from build123d import *

# Parameters (mm, degrees)
F0_W    = 7
F0_H    = 11
F0_W_2  = 5
F0_H_2  = 15
F0_W_3  = 20
F0_H_3  = 7
F2_SIZE = 1.99999


# Not quite as in the source:
# - a fillet or chamfer is up to 0.001 mm smaller than in the source, because OpenCascade refuses the exact size


with BuildPart() as f1:
    # F0 (on Front) → F1 (revolve)
    with BuildSketch(Plane.XZ):
        Polygon((33, 0), (0, 0), (0, -13), (33, -13), (33, -11), align=None)
        with Locations((36.5, -5.5)):
            Rectangle(F0_W, F0_H)
        Polygon((49, 0), (40, 0), (40, -11), (40, -17), (49, -17), (49, -15), align=None)
        with Locations((51.5, -7.5)):
            Rectangle(F0_W_2, F0_H_2)
        Polygon((63, 0), (54, 0), (54, -15), (54, -17), (63, -17), (63, -9), align=None)
        Polygon((95, 0), (63, 0), (63, -9), (95, -9), (95, -7), align=None)
        with Locations((105, -3.5)):
            Rectangle(F0_W_3, F0_H_3)
    revolve(axis=Axis((51.5, 0, 0), (1, 0, 0)))

    # F2 (size 2 in the source; OpenCascade refuses exactly that, so slightly less here)
    f2_edges = [f1.edges().sort_by_distance(p)[0] for p in [
        (0, 0, 13),
        (33, 0, 13),
        (16.5, 0, -13),
        (40, 0, 17),
        (49, 0, 17),
        (54, 0, 17),
        (63, 0, 17),
        (95, 0, 9),
        (115, 0, 7),
    ]]
    chamfer(f2_edges, length=F2_SIZE)


solid = f1.part
Could you check a few things on this model? Use its own coordinates, in mm. A direction names the side the tool comes from. Give positions to 0.01 mm unless a question says otherwise; leave off trailing zeros. Order: outer loops, then holes, each group sorted by start corner. A loop starts at its lowest first (then second) coordinate and runs counter-clockwise, first axis right, second up. Notation, with made-up numbers: (26, 48.25) - (73, 48.25) arc R19 cw to (73, 79.25) - close; hole circle Ø5 at (6.25, 40.5). An arc over 180 degrees is marked (long way). One line per item, written item: value. Start each with the question number.
1. Imagine slicing it at A-A on x = 104. List the corners of the cut face in (y, z) for me.
2. Imagine slicing it at B-B on x = 18. List the corners of the cut face in (y, z) for me, plus the area to 3 significant figures.
3. If I drill on probe 1 along X at (y, z) = (-7, 14.5); probe 2 along X at (y, z) = (9, 3.5); probe 3 along X at (y, z) = (15.5, -1.5), over which ranges is the centre line in solid material (lowest first)?
4. For P1, Ø6, axis at x = 57.5, z = 3.5, coming from the +Y side; P2, Ø10, axis at x = 24.5, z = 2.5, coming from the +Y side; P3, Ø6, axis at x = 60, y = 9.5, coming from the -Z side, each with a flat end and sliding along its axis, tell me the tip position at first contact or that it passes through.
5. For faces 1 (the face through (16.703, -7.91, 10.316)), 2 (the face through (78.21, 8.923, 1.172)), 3 (the face through (54.13, -14.77, 3.28)), which set-ups out of +Z, -Z, +X, -X, +Y, -Y let a thin tool reach every point of the face, with its end or its side?
Values:
1. outline: circle Ø14 at (0, 0)
2. outline: circle Ø26 at (0, 0)
2. area: 531 mm²
3. probe 1: 41.1 to 47.9, 55.1 to 61.9
3. probe 2: 0 to 63
3. probe 3: 40.57 to 48.43, 54.57 to 62.43
4. P1: y = 16.99
4. P2: y = 13
4. P3: z = -15.71
5. face 1: -X
5. face 2: +X
5. face 3: none
